Model file for the job. Use its own axes, mm. A direction names the side the tool comes from. Round coordinates to 2 decimals unless told otherwise and drop trailing zeros. Order: outer loops, then holes, each group sorted by start corner. A loop starts at its lowest first (then second) coordinate and runs counter-clockwise, first axis right, second up. Notation, with made-up numbers: (-30, -3) - (-20, -3) arc R26 cw to (-20, 34) - close; hole circle Ø6 at (27.5, 0.5). An arc over 180 degrees is marked (long way). Put each result on its own line as item: value. Start each with the question number.
Item 1: Saw through at A-A on x = 0. List the corners of the cut face in (y, z).
Item 2: Mould opens along Y. For faces 1 (the face through (0, 51, 13)), 2 (the face through (28.412, 50.341, 5.938)), 3 (the face through (48.33, 27.15, 5.92)), 4 (the face through (22, 41, 0)) say: pulls with the +Y half, pulls with the -Y half, needs draft (parallel to the pull), parting line crosses it, or undercut.
Item 3: Probe probe 1 along X at (y, z) = (26.25, 14.25); probe 2 along Y at (x, z) = (47.5, 11.25); probe 3 along Z at (x, y) = (0.5, 55). List the from-to ranges inside material, lowest first.
Item 4: Saw through at C-C on z = 14.25. List the corners of the cut face in (x, y).
Item 5: Which spindle directions (+Z, -Z, +X, -X, +Y, -Y) get a long thin tool onto all of the face, cutting with end or side? Do faces 5 (the face through (46.897, 26.701, 13.479)), 6 (the face through (46, 28, 12)). Say none if no direction does.
Item 6: Saw through at B-B on z = 5. List the corners of the cut face in (x, y).
Item 7: Pin check, flat tips, straight feed: pin 1 Ø4 at (x, z) = (8.5, 9) entering from -Y; pin 2 Ø3.5 at (x, y) = (0, 52.5) entering from -Z; pin 3 Ø5 at (x, z) = (40, 11) entering from +Y. Stop position of each tip, or through.
```python
from build123d import *

# Parameters (mm, degrees)
SKETCH_1_R          = 1.5
EXTRUDE_1_DEPTH     = 15
SKETCH_2_R          = 3
CUT_EXTRUDE_1_DEPTH = 12


with BuildPart() as part:
    # 草图1 → 凸台-拉伸1 (new body)
    with BuildSketch(Plane.XY):
        with BuildLine():
            ThreePointArc((42.286167935, 15.39090645), (22.5, 38.97114317), (-7.814167995, 44.316348886))
            Line((-7.814167995, 44.316348886), (-10.41889066, 59.088465181))
            ThreePointArc((-10.41889066, 59.088465181), (30, 51.961524227), (56.381557247, 20.5212086))
            Line((56.381557247, 20.5212086), (42.286167935, 15.39090645))
        make_face()
        with Locations((45.466333699, 26.25)):
            Circle(SKETCH_1_R, mode=Mode.SUBTRACT)
        with Locations((0, 52.5)):
            Circle(SKETCH_1_R, mode=Mode.SUBTRACT)
    extrude(amount=EXTRUDE_1_DEPTH)

    # 草图2 → 切除-拉伸1 (cut)
    with BuildSketch(Plane.XY):
        with Locations((0, 52.5)):
            Circle(SKETCH_2_R)
        with Locations((45.466333699, 26.25)):
            Circle(SKETCH_2_R)
    extrude(amount=CUT_EXTRUDE_1_DEPTH, mode=Mode.SUBTRACT)

    # 草图6 → 切除-旋转1 (revolve, cut)
    with BuildSketch(Plane(origin=(0, 0, 0), x_dir=(0, 0, 1), z_dir=(-0.9848077530122092, -0.1736481776669239, 0))):
        Polygon((0, 60), (0, 56.36802701), (15, 60), align=None)
    revolve(axis=Axis((0, 0, 0), (0, 0, -1)), mode=Mode.SUBTRACT)


solid = part.part
```
Results found:
1. outline: (45, 0) - (49.5, 0) - (49.5, 12) - (51, 12) - (51, 15) - (45, 15) - close; (54, 12) - (55.5, 12) - (55.5, 0) - (56.37, 0) - (60, 15) - (54, 15) - close
2. face 1: undercut
2. face 2: pulls with the +Y half
2. face 3: undercut
2. face 4: needs draft
3. probe 1: x = 36.55 to 43.97, 46.97 to 53.75
3. probe 2: y = 17.29 to 24.04, 28.46 to 35.15
3. probe 3: z = 12 to 15
4. outline: (-10.39, 58.91) - (-7.81, 44.32) arc R45 cw to (42.29, 15.39) - (56.21, 20.46) arc R59.82 ccw to start; hole circle Ø3 at (0, 52.5); hole circle Ø3 at (45.47, 26.25)
5. face 5: +Z, -Z
5. face 6: -Z
6. outline: (-10, 56.7) - (-7.81, 44.32) arc R45 cw to (42.29, 15.39) - (54.11, 19.69) arc R57.58 ccw to start; hole circle Ø6 at (0, 52.5); hole circle Ø6 at (45.47, 26.25)
7. pin 1: stops at y = 43.76
7. pin 2: stops at z = 12
7. pin 3: stops at y = 45.73
